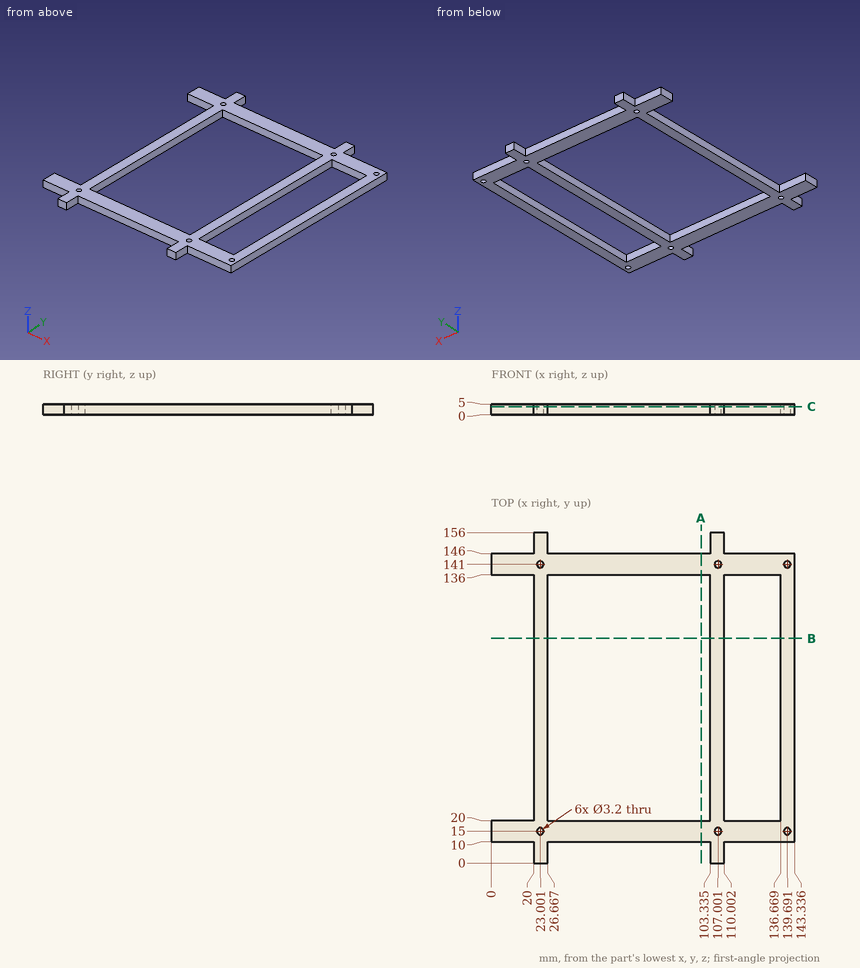
Geometry: see drawing. Coordinates: mm, zero at the bounding-box minimum. Give positions to 0.01 mm unless a question says otherwise; leave off trailing zeros. Order: outer loops, then holes, each group sorted by start corner. A loop starts at its lowest first (then second) coordinate and runs counter-clockwise, first axis right, second up.
Q1. Section B-B on y = 106. Output: boundary loops of the cut face in (x, z) (3 decimals), and give its area (3 significant figures).
Checked values:
outline: (20, 0) - (26.667, 0) - (26.667, 5) - (20, 5) - close; (103.335, 0) - (110.002, 0) - (110.002, 5) - (103.335, 5) - close; (136.669, 0) - (143.336, 0) - (143.336, 5) - (136.669, 5) - close
area: 100 mm2
Q2. Section A-A on x = 99. Output: boundary loops of the cut face in (y, z).
Checked values:
outline: (10, 0) - (20, 0) - (20, 5) - (10, 5) - close; (136, 0) - (146, 0) - (146, 5) - (136, 5) - close
Q3. Contact query for flat-ended pins moving along their axis: pin 1 Ø1.5 at (y, z) = (151.5, 2.5) entering from +X; pin 2 Ø1.5 at (x, z) = (10, 3.5) entering from -Y; pin 3 Ø3 at (y, z) = (54.5, 0.5) entering from -X; pin 4 Ø3.5 at (x, y) = (139.691, 15) entering from +Z. Output: stop coordinate, or through.
Checked values:
pin 1: stops at x = 110
pin 2: stops at y = 10
pin 3: stops at x = 20
pin 4: stops at z = 5
Q4. Section C-C on z = 3.8. State how many separate pieces and enclosed holes the cut face has, and give its area (3 significant figures).
Checked values:
separate pieces: 1
enclosed holes: 8
area: 5,410 mm2
Q5. Ray query, probe 1 along X at (y, z) = (112, 3.95) (3 decimals); probe 2 along X at (y, z) = (8.5, 0.35) (3 decimals); probe 3 along Y at (x, z) = (59, 2.3). Return the intervals inside material, ascending.
Checked values:
probe 1: x = 20 to 26.667, 103.335 to 110.002, 136.669 to 143.336
probe 2: x = 20 to 26.667, 103.335 to 110.002
probe 3: y = 10 to 20, 136 to 146
